Check sheet for the modelled part. Datum: model origin and axes. Units: mm. A direction names the side the tool comes from. Round coordinates to 2 decimals unless told otherwise and drop trailing zeros. Loops run counter-clockwise (first coordinate to the right, second up) from the corner with the lowest first, then second, coordinate; pieces in that order, holes last. Notation, with made-up numbers: M 72,-34 L 108,-34 A19 cw 108,-25 Z; hole C 12,-27.5 d7. An arc over 180 degrees is marked long. One line per question, with ' | ' between items. Start each with the question number.
(1) Tool access check on faces 1 (the face through (-28, 1, -22.9)), 2 (the face through (-1, 2.5, 0)), 3 (the face through (-7.076, 1, 24)). Record the directions out of +Z, -Z, +X, -X, +Y, -Y that give a thin tool (end or side, any length) a straight path to the whole face; none if there is none.
(2) Go/stop test with a flat-tipped pin: P1, Ø1.2, axis at x = -1, y = 1.5, coming from the +Z side. Record where the tip stops, or that it passes through.
(3) Section check B-B (x = -3). Record the boundary of the cut face in (y, z).
(4) Draft check along X on faces 4 (the face through (-14, 1, -25.4)), 5 (the face through (-49.53, 1, 0)), 6 (the face through (28, 1, -22.9)). Enter one of: +X half, -X half, draft (parallel to the pull), parting line (faces both ways), or undercut.
(5) Thickness scan on probe 1 along Z at (x, y) = (-23.5, 0.8). Record the ranges inside material, lowest first. Write a range as [from, to].
(6) Section check A-A (y = 1.15). Record the boundary of the cut face in (x, z), and give its area (3 significant figures).
```python
from build123d import *

# Parameters (mm, degrees)
SKETCH1_W           = 99.06
SKETCH1_H           = 50.8
BOSS_EXTRUDE1_DEPTH = 2.5
SKETCH2_W           = 14.151428572
SKETCH2_H           = 2.5
CUT_EXTRUDE1_DEPTH  = 2.54


with BuildPart() as part:
    # Sketch1 → Boss-Extrude1 (new body)
    with BuildSketch(Plane(origin=(0, 0, 0), x_dir=(1, 0, 0), z_dir=(0, 1, 0))):
        Rectangle(SKETCH1_W, SKETCH1_H)
    extrude(amount=BOSS_EXTRUDE1_DEPTH)

    # Sketch2 → Cut-Extrude1 (cut)
    with BuildSketch(Plane(origin=(0, 2.5, 0), x_dir=(1, 0, 0), z_dir=(0, 1, 0))):
        with Locations((-28.302857143, 24.15)):
            Rectangle(SKETCH2_W, SKETCH2_H)
        with Locations((0, 24.15)):
            Rectangle(SKETCH2_W, SKETCH2_H)
        with Locations((28.302857143, 24.15)):
            Rectangle(SKETCH2_W, SKETCH2_H)
        with Locations((-28.302857143, -24.15)):
            Rectangle(SKETCH2_W, SKETCH2_H)
        with Locations((0, -24.15)):
            Rectangle(SKETCH2_W, SKETCH2_H)
        with Locations((28.302857143, -24.15)):
            Rectangle(SKETCH2_W, SKETCH2_H)
    extrude(amount=-CUT_EXTRUDE1_DEPTH, mode=Mode.SUBTRACT)


solid = part.part
```
The answers:
1) face 1: -Z, +Y, -Y | face 2: +Z, -Z, +X, -X, +Y | face 3: +Z, +Y, -Y
2) P1: z = 22.9
3) outline: M 0,-22.9 L 2.5,-22.9 L 2.5,22.9 L 0,22.9 Z
4) face 4: draft | face 5: -X half | face 6: undercut
5) probe 1: [-22.9, 22.9]
6) outline: M -49.53,-25.4 L -35.38,-25.4 L -35.38,-22.9 L -21.23,-22.9 L -21.23,-25.4 L -7.08,-25.4 L -7.08,-22.9 L 7.08,-22.9 L 7.08,-25.4 L 21.23,-25.4 L 21.23,-22.9 L 35.38,-22.9 L 35.38,-25.4 L 49.53,-25.4 L 49.53,25.4 L 35.38,25.4 L 35.38,22.9 L 21.23,22.9 L 21.23,25.4 L 7.08,25.4 L 7.08,22.9 L -7.08,22.9 L -7.08,25.4 L -21.23,25.4 L -21.23,22.9 L -35.38,22.9 L -35.38,25.4 L -49.53,25.4 Z | area: 4,820 mm²
